For this review, use the dimensioned drawing (mm, ordinates from the lowest corner) and the shaded views. Coordinates: 2 decimals unless noted, no trailing zeros. Write each loop counter-clockwise with the first axis right and the second up, starting at its lowest first coordinate (ties: lowest second). Pieces come first, ordered by that corner, then holes. Notation, with made-up numbers: (29, 83.25) - (60, 83.25) arc R29 ccw to (60, 112.25) - close; hole circle Ø4 at (-30.5, 34.25). An arc over 180 degrees is marked (long way). Put each result on its own line as item: value.
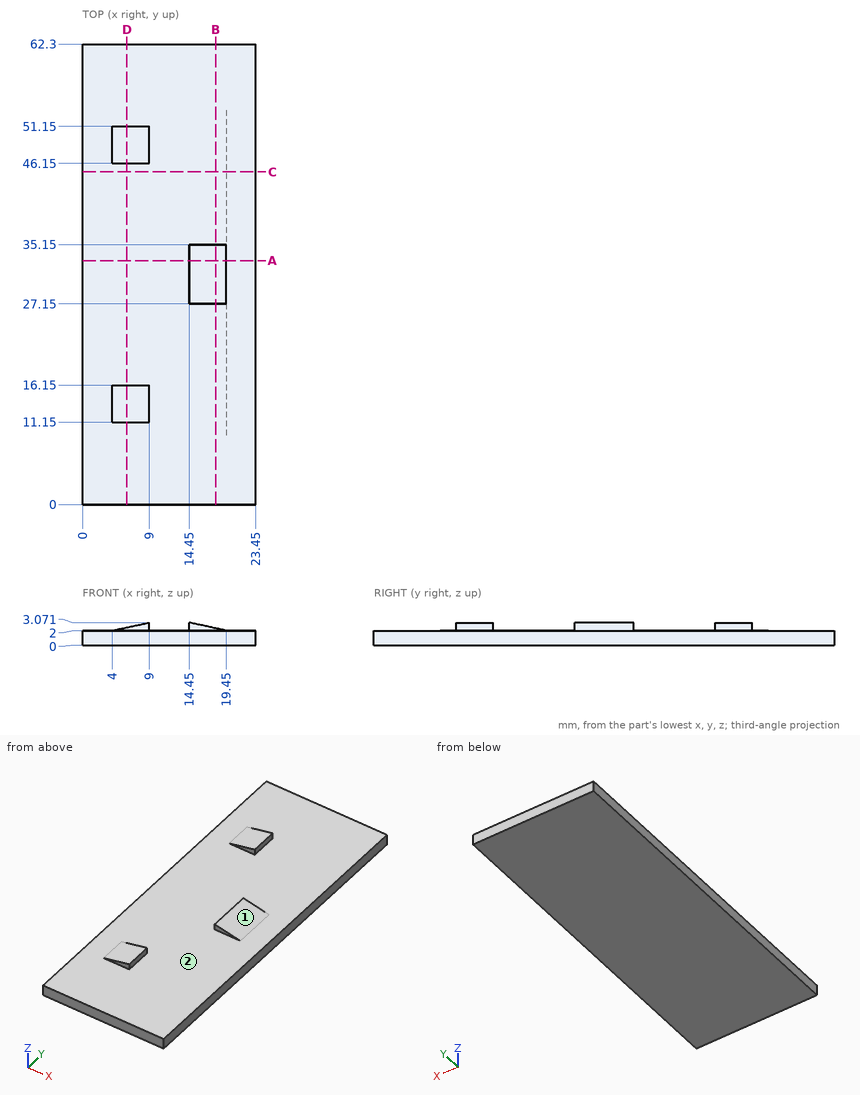
1. Consider section C-C on y = 45. State the section outline as (x, z) points.
Determined:
outline: (0, 0) - (23.45, 0) - (23.45, 2) - (0, 2) - close
2. Consider section D-D on x = 6. State the section outline as (y, z) points.
Determined:
outline: (0, 0) - (62.3, 0) - (62.3, 2) - (51.15, 2) - (51.15, 2.43) - (46.15, 2.43) - (46.15, 2) - (16.15, 2) - (16.15, 2.43) - (11.15, 2.43) - (11.15, 2) - (0, 2) - close
3. For pin 1 Ø0.5 at (x, z) = (7.5, 2.5) entering from -Y; pin 2 Ø1.2 at (x, z) = (6.5, 2.5) entering from +Y; pin 3 Ø1.2 at (x, z) = (16.5, 3) entering from -Y; pin 4 Ø4 at (x, y) = (3.5, 33) entering from +Z, all flat-tipped, find the tip position at first contact; note any pin that passes through.
Determined:
pin 1: stops at y = 11.15
pin 2: stops at y = 62.3
pin 3: stops at y = 27.15
pin 4: stops at z = 2
4. Consider section A-A on y = 33. State the section outline as (x, z) points.
Determined:
outline: (0, 0) - (23.45, 0) - (23.45, 2) - (19.45, 2) - (14.45, 3.07) - (14.45, 2) - (0, 2) - close
5. To check wall thickness, follow probe 1 along Y at (x, z) = (7, 2.2); probe 2 along Z at (x, y) = (9.75, 32.5); probe 3 along Z at (x, y) = (7.5, 16). State the ranges of each line that lie inside material, in increasing order.
Determined:
probe 1: y = 11.15 to 16.15, 46.15 to 51.15
probe 2: z = 0 to 2
probe 3: z = 0 to 2.75
6. The part is to be moulded in two halves that separate along Y. For the marked faces 1 and 2, say which applies: +Y half, -Y half, draft (parallel to the pull), parting line (faces both ways), or undercut.
Determined:
face 1: draft
face 2: undercut
7. Consider section B-B on x = 18. State the section outline as (y, z) points, plus the area to 3 significant figures.
Determined:
outline: (0, 0) - (62.3, 0) - (62.3, 2) - (35.15, 2) - (35.15, 2.31) - (27.15, 2.31) - (27.15, 2) - (0, 2) - close
area: 127 mm^2
